Part print with two shaded views. Sizes in mm from the minimum x, y, z corner. Round coordinates to 2 decimals unless told otherwise and drop trailing zeros. Write each loop counter-clockwise with the first axis right and the second up, starting at its lowest first coordinate (ties: lowest second). Pieces come first, ordered by that corner, then holes.
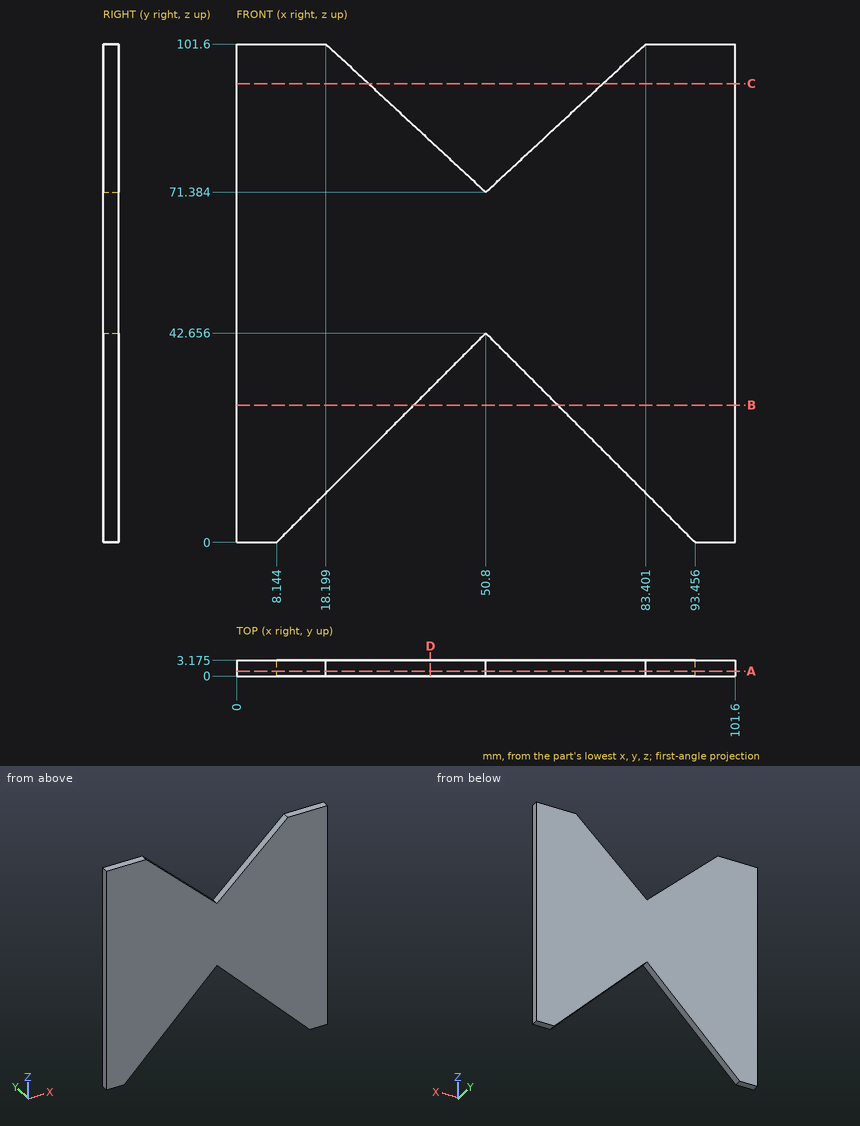
Q1. Cut at B-B on z = 28. Write the cut outline in (x, y) (1 decimal).
Values follow:
outline: (0, 0) - (36.1, 0) - (36.1, 3.2) - (0, 3.2) - close; (65.5, 0) - (101.6, 0) - (101.6, 3.2) - (65.5, 3.2) - close
Q2. Cut at A-A on y = 1. Write the cut outline in (x, z) (1 decimal).
Values follow:
outline: (0, 0) - (8.1, 0) - (50.8, 42.7) - (93.5, 0) - (101.6, 0) - (101.6, 101.6) - (83.4, 101.6) - (50.8, 71.4) - (18.2, 101.6) - (0, 101.6) - close
Q3. Wall check: L1, parallel to X at y = 1.2, z = 81 (1 decimal); L2, parallel to X at y = 3, z = 19.5 (1 decimal); L3, parallel to Z at x = 26.5, y = 0.9 (1 decimal). Give the ranges that are in metal, low to high.
Values follow:
L1: x = 0 to 40.4, 61.2 to 101.6
L2: x = 0 to 27.6, 74 to 101.6
L3: z = 18.4 to 93.9
Q4. Cut at C-C on z = 93.5. Write the cut outline in (x, y) (1 decimal).
Values follow:
outline: (0, 0) - (26.9, 0) - (26.9, 3.2) - (0, 3.2) - close; (74.7, 0) - (101.6, 0) - (101.6, 3.2) - (74.7, 3.2) - close
Q5. Cut at D-D on x = 39.5. Write the cut outline in (y, z) (1 decimal).
Values follow:
outline: (0, 31.4) - (3.2, 31.4) - (3.2, 81.9) - (0, 81.9) - close
